Model file for the job. Use its own axes, mm. A direction names the side the tool comes from. Give positions to 0.01 mm unless a question says otherwise; leave off trailing zeros. Write each loop counter-clockwise with the first axis right and the second up, starting at its lowest first coordinate (ties: lowest second). Pieces come first, ordered by that corner, then holes. Notation, with made-up numbers: (-38.75, 74) - (18.25, 74) arc R31 ccw to (18.25, 99) - close; hole circle Ø9 at (56.25, 77). An arc over 180 degrees is marked (long way). Use a Markdown table: item, result. Add a question column.
```python
from build123d import *

# Parameters (mm, degrees)
SKETCH1_W               = 13.8
SKETCH1_H               = 8.8
BOSS_EXTRUDE1_DEPTH     = 3
SKETCH2_W               = 2
SKETCH2_H               = 35
BOSS_EXTRUDE2_DEPTH     = 3
SKETCH3_W               = 1.2
SKETCH3_H               = 6
BOSS_EXTRUDE3_DEPTH     = 7
FILLET3_R               = 10
SKETCH5_W               = 15
SKETCH5_H               = 13.8
BOSS_EXTRUDE4_DEPTH     = 4
SKETCH6_R               = 1.5
CUT_EXTRUDE4_DEPTH      = 38.968539608
BOSS_EXTRUDE5_DEPTH     = 2
CHAMFER2_SIZE           = 3
BOSS_EXTRUDE7_DEPTH     = 1.2
SKETCH12_W              = 15
SKETCH12_H              = 4
BOSS_EXTRUDE8_DEPTH     = 3
SKETCH13_W              = 15
SKETCH13_H              = 4
BOSS_EXTRUDE9_DEPTH     = 3
CUT_EXTRUDE7_DEPTH      = 43.28486727
CUT_EXTRUDE7_DEPTH_BACK = 43.28486727
CUT_EXTRUDE8_DEPTH      = 43.28486727
CUT_EXTRUDE8_DEPTH_BACK = 43.28486727
SKETCH15_W              = 0.807911756
SKETCH15_H              = 0.64
CUT_EXTRUDE9_DEPTH      = 41.244591358
CUT_EXTRUDE9_DEPTH_BACK = 41.244591358
SKETCH16_W              = 0.64
SKETCH16_H              = 0.6
CHAMFER3_SIZE           = 1
SKETCH18_W              = 20.701942652
SKETCH18_H              = 41.728044518
CUT_EXTRUDE10_DEPTH     = 36
SKETCH19_W              = 11.097134513
SKETCH19_H              = 20.928514419
CUT_EXTRUDE11_DEPTH     = 3


# Some blends are built 0.0001 mm under size
with BuildPart() as part:
    # Sketch1 → Boss-Extrude1 (new body)
    with BuildSketch(Plane(origin=(0, 0, 0), x_dir=(0, 0, -1), z_dir=(1, 0, 0))):
        Rectangle(SKETCH1_W, SKETCH1_H)
    extrude(amount=BOSS_EXTRUDE1_DEPTH)

    # Sketch2 → Boss-Extrude2 (add)
    with BuildSketch(Plane(origin=(3, 0, 0), x_dir=(0, 0, -1), z_dir=(1, 0, 0))):
        with Locations((0, -13.1)):
            Rectangle(SKETCH2_W, SKETCH2_H)
    extrude(amount=BOSS_EXTRUDE2_DEPTH)

    # Sketch3 → Boss-Extrude3 (add)
    with BuildSketch(Plane(origin=(6, 0, 0), x_dir=(0, 0, -1), z_dir=(1, 0, 0))):
        with Locations((0, -27.6)):
            Rectangle(SKETCH3_W, SKETCH3_H)
    extrude(amount=BOSS_EXTRUDE3_DEPTH)

    # Fillet3
    # the kernel refuses this fillet: 10 mm, written as the material it adds along each edge
    with BuildSketch(Plane(origin=(3, -4.4, 1), x_dir=(-1, 0, 0), z_dir=(0, 0, -1))) as fillet3_piece_1:
        with BuildLine():
            CenterArc((10, -7.141428429), FILLET3_R, 134.427004001, 45.572995999)
            Line((0, -7.141428429), (0, 0))
            Line((0, 0), (3, 0))
        make_face()
    extrude(amount=2)

    # Sketch5 → Boss-Extrude4 (add)
    with BuildSketch(Plane(origin=(0, 4.4, 0), x_dir=(1, 0, 0), z_dir=(0, 1, 0))):
        with Locations((-4.5, 0)):
            Rectangle(SKETCH5_W, SKETCH5_H)
    extrude(amount=BOSS_EXTRUDE4_DEPTH)

    # Sketch6 → Cut-Extrude4 (cut, through all)
    with BuildSketch(Plane.XZ.offset(-4.4)):
        with Locations(Location((-6, 3, 0), (0, 0, 270))):
            Circle(SKETCH6_R)
        with Locations(Location((-6, -3, 0), (0, 0, 270))):
            Circle(SKETCH6_R)
    extrude(amount=-CUT_EXTRUDE4_DEPTH, mode=Mode.SUBTRACT)

    # Sketch8 → Boss-Extrude5 (add)
    with BuildSketch(Plane(origin=(0, 0, -1), x_dir=(-1, 0, 0), z_dir=(0, 0, -1))):
        Polygon((-3, -18.758153574), (0, -4.4), (-3, -4.4), align=None)
    extrude(amount=-BOSS_EXTRUDE5_DEPTH)

    # Chamfer2
    chamfer2_edges = [part.edges().sort_by_distance(p)[0] for p in [
        (3, 4.4, 0),
    ]]
    chamfer(chamfer2_edges, length=CHAMFER2_SIZE - 0.0001)  # a hair under: the kernel refuses the full size

    # Sketch11 → Boss-Extrude7 (add)
    with BuildSketch(Plane(origin=(0, 0, -0.6), x_dir=(-1, 0, 0), z_dir=(0, 0, -1))):
        Polygon((-6, -24.6), (-13, -24.6), (-6, 1.742521041), align=None)
    extrude(amount=-BOSS_EXTRUDE7_DEPTH)

    # Sketch12 → Boss-Extrude8 (add)
    with BuildSketch(Plane(origin=(0, 0, -6.9), x_dir=(-1, 0, 0), z_dir=(0, 0, -1))):
        with Locations((4.5, 6.4)):
            Rectangle(SKETCH12_W, SKETCH12_H)
    extrude(amount=BOSS_EXTRUDE8_DEPTH)

    # Sketch13 → Boss-Extrude9 (add)
    with BuildSketch(Plane.XY.offset(6.9)):
        with Locations((-4.5, 6.4)):
            Rectangle(SKETCH13_W, SKETCH13_H)
    extrude(amount=BOSS_EXTRUDE9_DEPTH)

    # Sketch14 → Cut-Extrude7 (cut, two sides: drawn at the far end of the back side and taken through both)
    with BuildSketch(Plane(origin=(0, 8.4, 0), x_dir=(1, 0, 0), z_dir=(0, 1, 0)).offset(-CUT_EXTRUDE7_DEPTH_BACK)):
        with BuildLine():
            Line((-7.5, 7), (-7.5, -7))
            ThreePointArc((-7.5, -7), (-6, -8.5), (-4.5, -7))
            Line((-4.5, -7), (-4.5, 7))
            ThreePointArc((-4.5, 7), (-6, 8.5), (-7.5, 7))
        make_face()
    extrude(amount=CUT_EXTRUDE7_DEPTH + CUT_EXTRUDE7_DEPTH_BACK, mode=Mode.SUBTRACT)

    # Sketch15 → Cut-Extrude8 (cut, two sides: drawn at the far end of the back side and taken through both)
    with BuildSketch(Plane.XZ.offset(30.6).offset(-CUT_EXTRUDE8_DEPTH_BACK)):
        with Locations((12.596044122, 0)):
            Rectangle(SKETCH15_W, SKETCH15_H)
    extrude(amount=CUT_EXTRUDE8_DEPTH + CUT_EXTRUDE8_DEPTH_BACK, mode=Mode.SUBTRACT)

    # Sketch16 → Cut-Extrude9 (cut, two sides: drawn at the far end of the back side and taken through both)
    with BuildSketch(Plane(origin=(12.192088244, 0, 0), x_dir=(0, 0, -1), z_dir=(1, 0, 0)).offset(-CUT_EXTRUDE9_DEPTH_BACK)):
        with Locations((0, -30.3)):
            Rectangle(SKETCH16_W, SKETCH16_H)
    extrude(amount=CUT_EXTRUDE9_DEPTH + CUT_EXTRUDE9_DEPTH_BACK, mode=Mode.SUBTRACT)

    # Chamfer3
    chamfer3_edges = [part.edges().sort_by_distance(p)[0] for p in [
        (12.192088244, -30, 0),
    ]]
    chamfer(chamfer3_edges, length=CHAMFER3_SIZE)

    # Sketch18 → Cut-Extrude10 (cut)
    with BuildSketch(Plane.XY.offset(9.9)):
        with Locations((9.448105839, -12.464022259)):
            Rectangle(SKETCH18_W, SKETCH18_H)
    extrude(amount=-CUT_EXTRUDE10_DEPTH, mode=Mode.SUBTRACT)

    # Sketch19 → Cut-Extrude11 (cut)
    with BuildSketch(Plane.XZ.offset(-4.4)):
        with Locations((-6.451432743, 0.56425721)):
            Rectangle(SKETCH19_W, SKETCH19_H)
    extrude(amount=-CUT_EXTRUDE11_DEPTH, mode=Mode.SUBTRACT)


solid = part.part
```
(1) Band-saw the part on A-A (x = -6). Write the cut outline in (y, z).
(2) Band-saw the part on B-B (y = 7.9). Write the cut outline in (x, z).
(3) Probe probe 1 along X at (y, z) = (8.15, 3.25); probe 2 along X at (y, z) = (8.1, 7.75); probe 3 along Z at (x, y) = (-5.75, 7.7). List the from-to ranges inside material, lowest first. Write a range as [from, to].
(4) Band-saw the part on C-C (z = -2.25). Write the cut outline in (x, y), then the cut area to 3 significant figures.
(5) Which spindle directions (+Z, -Z, +X, -X, +Y, -Y) get a long thin tool onto all of the face, cutting with end or side? Do faces 1 (the cylindrical face through (-6, 7.9, -8.5)), 2 (the flat face through (-8, 7.4, 0)). Say none if no direction does.
(6) Two-plate mould, pull along Z, no slides. Class faces 3 (the flat face through (-6, 8, -9.9)), 4 (the flat face through (-0.903, 8, 0)), 5 (the flat face through (-7.5, 8, 0)), 6 (the cylindrical face through (-6, 7.9, 8.5)): +Z half, -Z half, draft (parallel to the pull), parting line (faces both ways), or undercut.
Model answer:
| question | item | result |
|---|---|---|
| 1 | outline | (7.4, -9.9) - (8.4, -9.9) - (8.4, -8.5) - (7.4, -8.5) - close; (7.4, 8.5) - (8.4, 8.5) - (8.4, 9.9) - (7.4, 9.9) - close |
| 2 | outline | (-12, -9.9) - (-0.9, -9.9) - (-0.9, 9.9) - (-12, 9.9) - close; hole (-7.5, -7) arc R1.5 ccw to (-4.5, -7) - (-4.5, 7) arc R1.5 ccw to (-7.5, 7) - close |
| 3 | probe 1 | x = [-12, -7.5], [-4.5, -0.9] |
| 3 | probe 2 | x = [-12, -7.3], [-4.7, -0.9] |
| 3 | probe 3 | z = [-9.9, -8.48], [8.48, 9.9] |
| 4 | outline | (-12, 7.4) - (-7.5, 7.4) - (-7.5, 8.4) - (-12, 8.4) - close; (-4.5, 7.4) - (-0.9, 7.4) - (-0.9, 8.4) - (-4.5, 8.4) - close |
| 4 | area | 8.10 mm^2 |
| 5 | face 1 | +Y, -Y |
| 5 | face 2 | +Z, -Z, +X, -X, -Y |
| 6 | face 3 | -Z half |
| 6 | face 4 | draft |
| 6 | face 5 | undercut |
| 6 | face 6 | undercut |
